Verification items for this drawing (mm, ordinates from the low corner). Round coordinates to 2 decimals unless told otherwise and drop trailing zeros. Order: outer loops, then holes, each group sorted by start corner. A loop starts at its lowest first (then second) coordinate and runs counter-clockwise, first axis right, second up. Notation, with made-up numbers: (52.5, -22.5) -> (83.5, -22.5) arc R16 ccw to (83.5, -9.5) -> close; hole circle Ø8 at (56, 76.5). An arc over 180 degrees is marked (long way). Answer in a Markdown table with one row per item. Add a question column.
1. Draft check along Z on the marked faces 1, 2, 3 and 4. Enter one of: +Z half, -Z half, draft (parallel to the pull), parting line (faces both ways), or undercut.
2. Sectioned sample at D-D, the plane x = 12.5. Record the boundary of the cut face in (y, z), then the cut area to 3 significant figures.
3. Depth check by flat-ended pin: P1, Ø4.5, axis at x = 11.43, z = 17.5, coming from the +Y side. Enter the tip coordinate at first touch or a pass-through.
4. Sectioned sample at A-A, the plane x = 4.5. Record the boundary of the cut face in (y, z).
5. Sectioned sample at B-B, the plane y = 1.65. Record the boundary of the cut face in (x, z).
6. Material ranges on L1, parallel to Z at x = 4.5, y = 2.8; L2, parallel to Z at x = 13, y = 1.4 (1 decimal); L3, parallel to X at y = 2.6, z = 18.25 (1 decimal), recorded low to high. Write a range as from..to.
7. Sectioned sample at C-C, the plane z = 5.5. Record the boundary of the cut face in (x, y) (1 decimal).
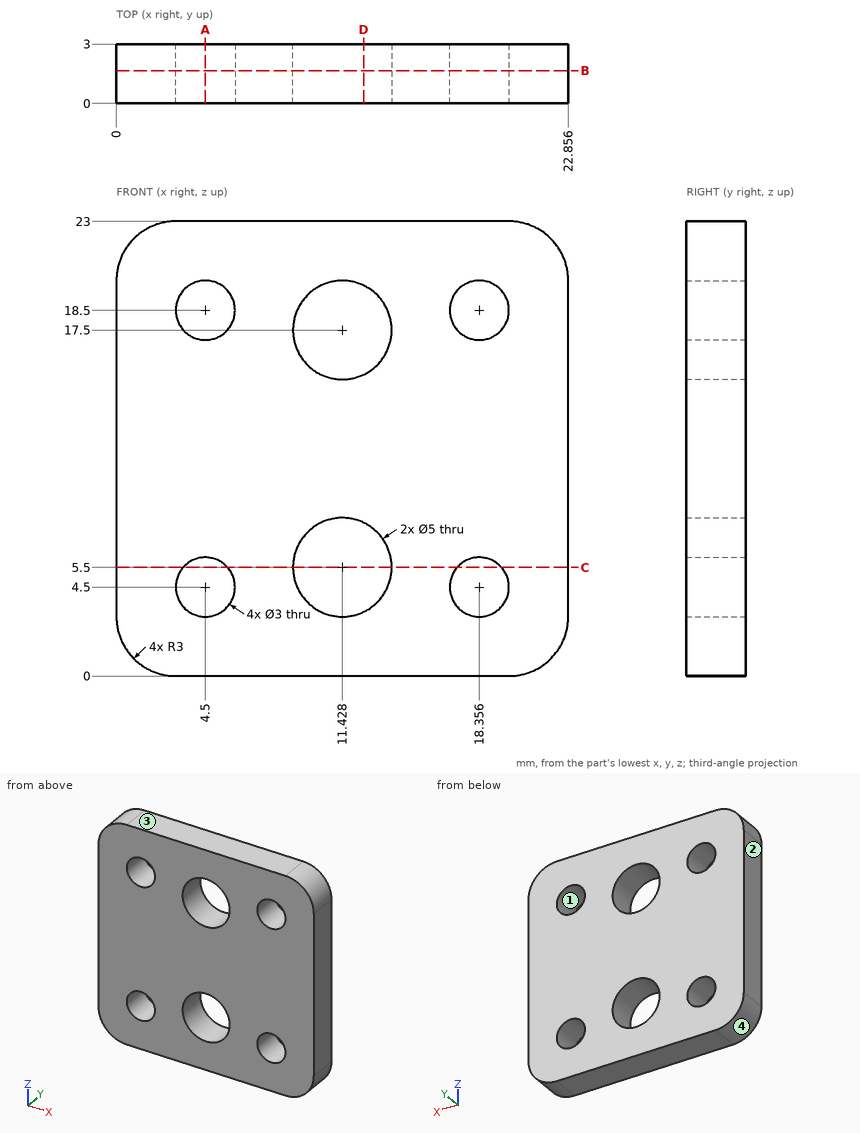
Answer key:
| question | item | result |
|---|---|---|
| 1 | face 1 | undercut |
| 1 | face 2 | draft |
| 1 | face 3 | +Z half |
| 1 | face 4 | -Z half |
| 2 | outline | (0, 0) -> (3, 0) -> (3, 3.24) -> (0, 3.24) -> close; (0, 7.76) -> (3, 7.76) -> (3, 15.24) -> (0, 15.24) -> close; (0, 19.76) -> (3, 19.76) -> (3, 23) -> (0, 23) -> close |
| 2 | area | 41.9 mm² |
| 3 | P1 | passes through |
| 4 | outline | (0, 0) -> (3, 0) -> (3, 3) -> (0, 3) -> close; (0, 6) -> (3, 6) -> (3, 17) -> (0, 17) -> close; (0, 20) -> (3, 20) -> (3, 23) -> (0, 23) -> close |
| 5 | outline | (0, 3) arc R3 ccw to (3, 0) -> (19.86, 0) arc R3 ccw to (22.86, 3) -> (22.86, 20) arc R3 ccw to (19.86, 23) -> (3, 23) arc R3 ccw to (0, 20) -> close; hole circle Ø3 at (4.5, 4.5); hole circle Ø3 at (4.5, 18.5); hole circle Ø5 at (11.43, 5.5); hole circle Ø5 at (11.43, 17.5); hole circle Ø3 at (18.36, 4.5); hole circle Ø3 at (18.36, 18.5) |
| 6 | L1 | z = 0..3, 6..17, 20..23 |
| 6 | L2 | z = 0..3.6, 7.4..15.6, 19.4..23 |
| 6 | L3 | x = 0..3, 6..9, 13.8..16.9, 19.8..22.9 |
| 7 | outline | (0, 0) -> (3.4, 0) -> (3.4, 3) -> (0, 3) -> close; (5.6, 0) -> (8.9, 0) -> (8.9, 3) -> (5.6, 3) -> close; (13.9, 0) -> (17.2, 0) -> (17.2, 3) -> (13.9, 3) -> close; (19.5, 0) -> (22.9, 0) -> (22.9, 3) -> (19.5, 3) -> close |
